from build123d import *

# Parameters (mm, degrees)
SKETCH001_W       = 110
SKETCH001_H       = 120
PAD005_DEPTH      = 44
SKETCH002_W       = 102
SKETCH002_H       = 112
POCKET002_DEPTH   = 6
SKETCH010_R       = 2
SKETCH010_W       = 80
SKETCH010_H       = 101
SKETCH010_W_2     = 96
SKETCH010_H_2     = 15.5
POCKET003_DEPTH   = 10
SKETCH011_W       = 96
SKETCH011_H       = 85
POCKET004_DEPTH   = 7
SKETCH012_W       = 102
SKETCH012_H       = 112
POCKET005_DEPTH   = 25
SKETCH014_W       = 55
SKETCH014_H       = 30
PAD006_DEPTH      = 9
SKETCH013_W       = 50
SKETCH013_H       = 15
POCKET006_DEPTH   = 9
FILLET_R          = 5
SKETCH015_R       = 2
POCKET007_DEPTH   = 6
CYLINDER003_R     = 3.6
CYLINDER003_DEPTH = 5
CYLINDER004_R     = 10
CYLINDER004_DEPTH = 16
SKETCH016_R       = 5.5
SKETCH016_R_2     = 1.125
POCKET008_DEPTH   = 4


with BuildPart() as part:
    # Sketch001 → Pad005 (new body)
    with BuildSketch(Plane.XY):
        with Locations((0, -10)):
            Rectangle(SKETCH001_W, SKETCH001_H)
    extrude(amount=PAD005_DEPTH)

    # Sketch002 (on Face5 of Pad005) → Pocket002 (cut)
    with BuildSketch(Plane(origin=(0, 0, 0), x_dir=(1, 0, 0), z_dir=(0, 0, -1))):
        with Locations((0, 10)):
            Rectangle(SKETCH002_W, SKETCH002_H)
    extrude(amount=-POCKET002_DEPTH, mode=Mode.SUBTRACT)

    # Sketch010 (on Face11 of Pocket002) → Pocket003 (cut)
    with BuildSketch(Plane(origin=(0, 0, 6), x_dir=(1, 0, 0), z_dir=(0, 0, -1))):
        with Locations((-45, 57)):
            Circle(SKETCH010_R)
        with Locations((45, 57)):
            Circle(SKETCH010_R)
        with Locations((45, -40.5)):
            Circle(SKETCH010_R)
        with Locations((-45, -40.5)):
            Circle(SKETCH010_R)
        with Locations((0, 10.5)):
            Rectangle(SKETCH010_W, SKETCH010_H)
        with Locations((0, 42.25)):
            Rectangle(SKETCH010_W_2, SKETCH010_H_2)
    extrude(amount=-POCKET003_DEPTH, mode=Mode.SUBTRACT)

    # Sketch011 → Pocket004 (cut)
    with BuildSketch(Plane.XY.offset(9)):
        with Locations((0, -7.5)):
            Rectangle(SKETCH011_W, SKETCH011_H)
    extrude(amount=POCKET004_DEPTH, mode=Mode.SUBTRACT)

    # Sketch012 → Pocket005 (cut)
    with BuildSketch(Plane.XY.offset(15)):
        with Locations((0, -10)):
            Rectangle(SKETCH012_W, SKETCH012_H)
    extrude(amount=POCKET005_DEPTH, mode=Mode.SUBTRACT)

    # Sketch014 (on Face5 of Pocket005) → Pad006 (join)
    with BuildSketch(Plane.XY.offset(44)):
        with Locations((-27.5, -55)):
            Rectangle(SKETCH014_W, SKETCH014_H)
    extrude(amount=-PAD006_DEPTH)

    # Sketch013 (on Face5 of Pocket005) → Pocket006 (cut)
    with BuildSketch(Plane.XY.offset(44)):
        with Locations((-30, -62.5)):
            Rectangle(SKETCH013_W, SKETCH013_H)
    extrude(amount=-POCKET006_DEPTH, mode=Mode.SUBTRACT)

    # Fillet
    fillet_edges = [part.edges().sort_by_distance(p)[0] for p in [
        (55, -10, 44),
        (25, -70, 44),
        (-5, -62.5, 44),
        (-30, -55, 44),
        (-55, -2.5, 44),
        (0, 50, 44),
        (-55, 50, 22),
        (-55, -70, 17.5),
        (55, -70, 22),
        (55, 50, 22),
    ]]
    fillet(fillet_edges, radius=FILLET_R)

    # Sketch015 (on Face26 of Fillet) → Pocket007 (cut)
    with BuildSketch(Plane(origin=(0, 0, 35), x_dir=(1, 0, 0), z_dir=(0, 0, -1))):
        with Locations((-7, 45)):
            Circle(SKETCH015_R)
        with Locations((-32, 45)):
            Circle(SKETCH015_R)
    extrude(amount=-POCKET007_DEPTH, mode=Mode.SUBTRACT)

    # Cylinder003 → Cylinder003 (cut)
    with BuildSketch(Plane(origin=(0, -61, 15), x_dir=(1, 0, 0), z_dir=(0, -1, 0))):
        Circle(CYLINDER003_R)
    extrude(amount=CYLINDER003_DEPTH, mode=Mode.SUBTRACT)

    # Cylinder004 → Cylinder004 (cut)
    with BuildSketch(Plane(origin=(-33, -50, 19), x_dir=(1, 0, 0), z_dir=(0, -1, 0))):
        Circle(CYLINDER004_R)
    extrude(amount=CYLINDER004_DEPTH, mode=Mode.SUBTRACT)

    # Sketch016 (on Face6 of Pocket007) → Pocket008 (cut)
    with BuildSketch(Plane.XZ.offset(70)):
        with Locations((-7, 21.9)):
            Circle(SKETCH016_R)
        with Locations((7, 21.9)):
            Circle(SKETCH016_R)
        with Locations((0, 28.75)):
            Circle(SKETCH016_R_2)
        with Locations((0, 15)):
            Circle(SKETCH016_R_2)
        with Locations((-33, 19)):
            Circle(SKETCH016_R)
    extrude(amount=-POCKET008_DEPTH, mode=Mode.SUBTRACT)


solid = part.part
Geometry: final body of the model. Coordinates: model frame, mm. A direction names the side the tool comes from. Coordinates: 2 decimals unless noted, no trailing zeros. Order: outer loops, then holes, each group sorted by start corner. A loop starts at its lowest first (then second) coordinate and runs counter-clockwise, first axis right, second up.
(1) Access query for faces 1 (the face through (53, -9, 43)), 2 (the face through (-1, -9, 40)), 3 (the face through (44, -50, 10)). Directions: +Z, -Z, +X, -X, +Y, -Y. A direction counts if a zero-diameter tool reaches every point of the face in a straight line with its end or side. Return the directions, or none.
(2) Section query D-D (x = 45). Return the cut outline in (y, z), plus the area to 3 significant figures.
(3) First-contact query: pin 1 (21 mm diameter, centred on x = -29, y = -51.5, fed in from -Z). Flat tip, straight axial feed; report the tip coordinate or a pass-through.
(4) Section query B-B (y = -57). State how many separate pieces and enclosed holes the cut face has, plus the area to 3 significant figures.
(5) Material intervals for probe 1 along X at (y, z) = (-57, 8.25); probe 2 along Y at (x, z) = (-45, 10); probe 3 along Y at (x, z) = (-45, 8.5), sorted ascending.
(6) Draft query along Y for faces 4 (the face through (-54, -4, 42)), 5 (the face through (23, -69, 42)), 6 (the face through (44, 1, 9)). Return one class per face: pulls with the +Y half, pulls with the -Y half, needs draft (parallel to the pull), parting line crosses it, or undercut.
(7) Section query A-A (x = 7). Return the cut outline in (y, z).
Solution:
1. face 1: +Z, +X, +Y, -Y
1. face 2: none
1. face 3: -Z
2. outline: (-70, 0) - (-66, 0) - (-66, 6) - (-59, 6) - (-59, 15) - (-66, 15) - (-66, 40) - (46, 40) - (46, 15) - (42.5, 15) - (42.5, 6) - (46, 6) - (46, 0) - (50, 0) - (50, 39) arc R5 ccw to (45, 44) - (-65, 44) arc R5 ccw to (-70, 39) - close; (-55, 6) - (-50, 6) - (-50, 15) - (-55, 15) - close; (-34.5, 6) - (38.5, 6) - (38.5, 15) - (35, 15) - (35, 9) - (-34.5, 9) - close
2. area: 1,170 mm2
3. pin 1: stops at z = 6
4. separate pieces: 4
4. enclosed holes: 0
4. area: 676 mm2
5. probe 1: x = -55 to -47, -43 to -40, 40 to 43, 47 to 55
5. probe 2: y = -70 to -59, -55 to -50, 35 to 38.5, 42.5 to 50
5. probe 3: y = -70 to -59, -55 to -50, -34.5 to 38.5, 42.5 to 50
6. face 4: needs draft
6. face 5: pulls with the -Y half
6. face 6: undercut
7. outline: (-70, 0) - (-66, 0) - (-66, 6) - (-61, 6) - (-61, 15) - (-66, 15) - (-66, 16.4) - (-70, 16.4) - close; (-70, 27.4) - (-66, 27.4) - (-66, 40) - (46, 40) - (46, 15) - (40, 15) - (40, 6) - (46, 6) - (46, 0) - (50, 0) - (50, 39) arc R5 ccw to (45, 44) - (-65, 44) arc R5 ccw to (-70, 39) - close
